For this review, take the finished solid that the model builds, in its own axes (mm). A direction names the side the tool comes from. Coordinates: 2 decimals unless noted, no trailing zeros. Write each loop counter-clockwise with the first axis right and the second up, starting at its lowest first coordinate (ties: lowest second). Pieces come first, ordered by that corner, then holes. Notation, with made-up numbers: (14.5, 51.5) -> (59.5, 51.5) arc R21 ccw to (59.5, 71.5) -> close; hole circle Ø10 at (-6, 23.5). An arc over 180 degrees is marked (long way). Put each result on its own line as item: value. Start each with the question number.
Item 1: To check wall thickness, follow L1, parallel to X at y = -0.5, z = 0.6; L2, parallel to X at y = 1.7, z = -0.3; L3, parallel to Z at x = 8.5, y = 0.6. State the ranges of each line that lie inside material, in increasing order.
Item 2: Consider section A-A on x = 1.5. Give the boundary of the cut face in (y, z), and give its area (3 significant figures).
Item 3: For faces 4 (the flat face through (-1.41, -0.5, -0.86)), 5 (the flat face through (10, 0, 0)), list the 3-axis set-ups (+Z, -Z, +X, -X, +Y, -Y) from which the entire face can be reached by the end or side of a thin tool; tool diameter is ignored.
Item 4: Insertion check: P1, Ø2, axis at x = 1.5, z = -0.5, coming from the +Y side; P2, Ø0.9, axis at x = -1, z = 0, coming from the -Y side; P3, Ø1, axis at x = 7.5, y = 0, coming from the -Z side. Each pin has a flat end and moves straight along its axis. Give the tip position at first contact, or say it passes through.
Item 5: The part is to be moulded in two halves that separate along Y. For faces 1 (the cylindrical face through (4.93, -1.5, -0.07)), 2 (the flat face through (0, 2, 0)), 3 (the flat face through (-0.6, 0, 0)), say which applies: +Y half, -Y half, draft (parallel to the pull), parting line (faces both ways), or undercut.
Autodesk Inventor part; units mm, degrees
ref_plane "YZ Plane" through (0, 0, 0) normal (1, 0, 0) x (0, 1, 0)
ref_plane "XZ Plane" through (0, 0, 0) normal (0, 1, 0) x (-1, 0, 0)
ref_plane "XY Plane" through (0, 0, 0) normal (0, 0, 1) x (1, 0, 0)
sketch "スケッチ1" plane through (0, 0, 0) normal (0, 0, 1) x (1, 0, 0)
  line L0 (0, 0) -> (10, 0)
  line L1 (10, 0) -> (10, 1.5)
  line L2 (10, 1.5) -> (0, 1.5)
  line L3 (0, 1.5) -> (0, 0)
  line L4 (0, 0) -> (0, 2.75)
  line L5 (0, 0) -> (-2, 0)
  line L6 (-2, 0) -> (0, 0)
  line L7 (-2, 0) -> (-2, 1.15)
  arc A0 (0, 2.75) -> (-2, 1.15) centre (-0.0403, 0.7504) ccw
  dimension "d0" = 1.5
  dimension "d1" = 10
  dimension "d3" = 2
  dimension "d4" = 2.75
  dimension "d5" = 1.15
  dimension "d6" = 2
revolve "回転1" add sketch "スケッチ1" angle 360 about axis through (-2, 0, 0) along (1, 0, 0)
thread "ねじ1"
sketch "スケッチ2" plane through (-2, 0, 0) normal (-1, 0, 0) x (0, 0, 1)
  circle A0 centre (0, 0) radius 1.15
  line L0 (-0.575, 0.9959) -> (0.575, 0.9959)
  line L1 (0.575, 0.9959) -> (1.15, 0)
  line L2 (1.15, 0) -> (0.575, -0.9959)
  line L3 (0.575, -0.9959) -> (-0.575, -0.9959)
  line L4 (-0.575, -0.9959) -> (-1.15, 0)
  line L5 (-1.15, 0) -> (-0.575, 0.9959)
  dimension "d10" = 1.15
  dimension "d11" = 1.9919
extrude "押し出し1" cut sketch "スケッチ2" against normal blind 1.4 contours L2 L3 L4 L5 L0 L1
fillet "フィレット1" radius 0.2 6 edges at (-0.6, 0.9959, 0) (-0.6, 0.498, 0.8625) (-0.6, 0.498, -0.8625) (-0.6, -0.498, -0.8625) (-0.6, -0.9959, 0) (-0.6, -0.498, 0.8625)
fillet "フィレット2" radius 0.1 1 edges at (0, -1.5, 0)
fillet "フィレット3" radius 0.1 1 edges at (10, -1.5, 0)
properties part number "ネジボタンM3L10" material "鋼"
Return value:
1. L1: -0.6 to 10
1. L2: -1.79 to 0
1. L3: -1.37 to 1.37
2. outline: circle Ø3 at (0, 0)
2. area: 7.07 mm^2
3. face 4: -X
3. face 5: +Z, -Z, +X, +Y, -Y
4. P1: y = 1.5
4. P2: y = -2.68
4. P3: z = -1.5
5. face 1: parting line
5. face 2: draft
5. face 3: undercut
